Part model, mm, in its own coordinate system. Face numbers are marked on the shaded views. A direction names the side the tool comes from. Give positions to 0.01 mm unless a question says otherwise; leave off trailing zeros. Write each loop counter-clockwise with the first axis right and the second up, starting at its lowest first coordinate (ties: lowest second). Pieces come first, ordered by that corner, then holes. Notation, with made-up numbers: (10.25, 4) - (48.25, 4) arc R20 ccw to (48.25, 35) - close; hole circle Ø10 at (67, 3.5). An arc over 180 degrees is marked (long way). Answer in a Markdown table with one row per item. Add a question column.
1. Band-saw the part on C-C on y = 9. Write the cut outline in (x, z).
2. Band-saw the part on B-B on x = 0. Write the cut outline in (y, z), plus the area to 3 significant figures.
3. Which spindle directions (+Z, -Z, +X, -X, +Y, -Y) get a long thin tool onto all of the face, cutting with end or side? Do the marked faces 4 and 5. Say none if no direction does.
4. Drop a flat-ended pin along its axis: pin 1 Ø18.5 at (x, z) = (0, 14) entering from +Y. Give the stop position or say it passes through.
5. Pull direction Y, two halves, no side cores. Call the marked faces 1, 2 and 3: released by +Y, released by -Y, zero draft, split by the parting line, or undercut.
6. Probe line 1 along Z through (x, y) = (0, 34.4); line 2 along X through (y, z) = (26, 4.5). List the from-to ranges inside material, lowest first.
7. Band-saw the part on A-A on z = 14. Write the cut outline in (x, y), plus the area to 3 significant figures.
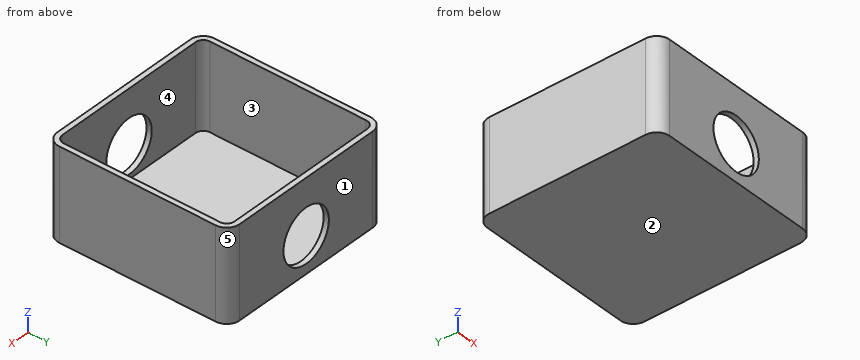
```python
from build123d import *

# Parameters (mm, degrees)
AUFSATZ_LINEAR_AUSTRAGEN1_DEPTH = 35
WANDUNG1_T                      = -2
SKIZZE2_R                       = 10.25
SCHNITT_LINEAR_AUSTRAGEN1_DEPTH = 71


with BuildPart() as part:
    # Skizze1 → Aufsatz-Linear austragen1 (new body)
    with BuildSketch(Plane.XY):
        with BuildLine():
            Line((-30, -35), (30, -35))
            ThreePointArc((30, -35), (33.535533906, -33.535533906), (35, -30))
            Line((35, -30), (35, 30))
            ThreePointArc((35, 30), (33.535533906, 33.535533906), (30, 35))
            Line((30, 35), (-30, 35))
            ThreePointArc((-30, 35), (-33.535533906, 33.535533906), (-35, 30))
            Line((-35, 30), (-35, -30))
            ThreePointArc((-35, -30), (-33.535533906, -33.535533906), (-30, -35))
        make_face()
    extrude(amount=AUFSATZ_LINEAR_AUSTRAGEN1_DEPTH)

    # Wandung1
    wandung1_openings = [part.faces().sort_by_distance(p)[0] for p in [
        (0, 0, 35),
    ]]
    offset(amount=WANDUNG1_T, openings=wandung1_openings, kind=Kind.INTERSECTION)

    # Skizze2 → Schnitt-Linear austragen1 (cut, through all)
    with BuildSketch(Plane.XZ.offset(35)):
        with Locations((0, 14)):
            Circle(SKIZZE2_R)
    extrude(amount=-SCHNITT_LINEAR_AUSTRAGEN1_DEPTH, mode=Mode.SUBTRACT)


solid = part.part
```
Values:
| question | item | result |
|---|---|---|
| 1 | outline | (-35, 0) - (35, 0) - (35, 35) - (33, 35) - (33, 2) - (-33, 2) - (-33, 35) - (-35, 35) - close |
| 2 | outline | (-35, 0) - (35, 0) - (35, 3.75) - (33, 3.75) - (33, 2) - (-33, 2) - (-33, 3.75) - (-35, 3.75) - close; (-35, 24.25) - (-33, 24.25) - (-33, 35) - (-35, 35) - close; (33, 24.25) - (35, 24.25) - (35, 35) - (33, 35) - close |
| 2 | area | 190 mm² |
| 3 | face 4 | +Z |
| 3 | face 5 | +Z, -Z, +X, +Y |
| 4 | pin 1 | passes through |
| 5 | face 1 | released by +Y |
| 5 | face 2 | zero draft |
| 5 | face 3 | undercut |
| 6 | line 1 | z = 0 to 3.75, 24.25 to 35 |
| 6 | line 2 | x = -35 to -33, 33 to 35 |
| 7 | outline | (-35, -30) arc R5 ccw to (-30, -35) - (-10.25, -35) - (-10.25, -33) - (-30, -33) arc R3 cw to (-33, -30) - (-33, 30) arc R3 cw to (-30, 33) - (-10.25, 33) - (-10.25, 35) - (-30, 35) arc R5 ccw to (-35, 30) - close; (10.25, -35) - (30, -35) arc R5 ccw to (35, -30) - (35, 30) arc R5 ccw to (30, 35) - (10.25, 35) - (10.25, 33) - (30, 33) arc R3 cw to (33, 30) - (33, -30) arc R3 cw to (30, -33) - (10.25, -33) - close |
| 7 | area | 448 mm² |
